Build history of the part. All positions in model axes, mm. Coordinates: 2 decimals unless noted, no trailing zeros. Loops run counter-clockwise (first coordinate to the right, second up) from the corner with the lowest first, then second, coordinate; pieces in that order, holes last. Notation, with made-up numbers: (24, -29.5) - (71, -29.5) arc R25 ccw to (71, 9.5) - close; hole circle Ø5 at (-21.75, 13). An arc over 180 degrees is marked (long way). One line per item, written item: value.
Autodesk Inventor part; units mm, degrees
ref_plane "YZ Plane" through (0, 0, 0) normal (1, 0, 0) x (0, 1, 0)
ref_plane "XZ Plane" through (0, 0, 0) normal (0, 1, 0) x (-1, 0, 0)
ref_plane "XY Plane" through (0, 0, 0) normal (0, 0, 1) x (1, 0, 0)
sketch "Sketch1" plane through (0, 0, 0) normal (1, 0, 0) x (0, 1, 0)
  line L0 (0, 0) -> (50.8, 0)
  line L1 (50.8, 0) -> (50.8, 76.2)
  line L2 (50.8, 76.2) -> (0, 76.2)
  line L3 (0, 76.2) -> (0, 0)
  dimension "d0" = 76.2
  dimension "d1" = 50.8
extrude "Extrusion1" add sketch "Sketch1" along normal blind 44.45
sketch "Sketch2" plane through (44.45, 0, 0) normal (1, 0, 0) x (0, 0, -1)
  line L0 (0, 50.8) -> (-76.2, 50.8)
  line L1 (-76.2, 50.8) -> (-76.2, 0)
  circle A0 centre (-17.272, 25.4) radius 6.35
  dimension "d4" = 12.7
  dimension "d5" = 25.4
  dimension "d6" = 58.928
extrude "Extrusion2" cut sketch "Sketch2" against normal blind 38.1
sketch "Sketch3" plane through (0, 0, 0) normal (0, 0, -1) x (-1, 0, 0)
  line L0 (0, 0) -> (0, 50.8)
  line L1 (0, 50.8) -> (-44.45, 50.8)
  line L2 (-44.45, 0) -> (-44.45, 50.8)
  line L3 (0, 0) -> (-44.45, 0)
  point P0 (-38.1, 44.45)
  point P1 (-12.7, 44.45)
  point P2 (-12.7, 6.35)
  point P3 (-38.1, 6.35)
  dimension "d9" = 6.35
  dimension "d10" = 6.35
  dimension "d11" = 6.35
  dimension "d12" = 12.7
  dimension "d13" = 12.7
  dimension "d14" = 6.35
  dimension "d15" = 6.35
  dimension "d16" = 6.35
hole "Hole1" at (38.1, 44.45, 0) at (12.7, 44.45, 0) at (12.7, 6.35, 0) at (38.1, 6.35, 0) direction (0, 0, 1) diameter 6.35 end through all
properties part number "Linear Bearing"
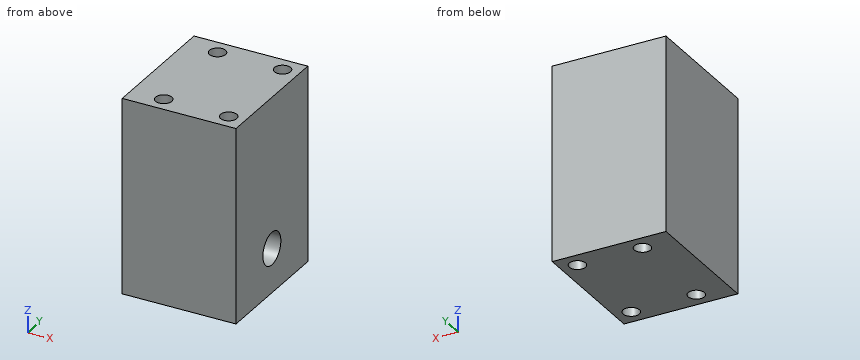
Item 1: Cut at B-B, the plane z = 47. Write the cut outline in (x, y) (3 decimals), then the cut area to 3 significant figures.
Check result:
outline: (0, 0) - (44.45, 0) - (44.45, 50.8) - (0, 50.8) - close; hole circle Ø6.35 at (12.7, 6.35); hole circle Ø6.35 at (12.7, 44.45); hole circle Ø6.35 at (38.1, 6.35); hole circle Ø6.35 at (38.1, 44.45)
area: 2,130 mm^2
Item 2: Cut at C-C, the plane y = 44.45. Write the cut outline in (x, z) (3 decimals), then the cut area to 3 significant figures.
Check result:
outline: (0, 0) - (9.525, 0) - (9.525, 76.2) - (0, 76.2) - close; (15.875, 0) - (34.925, 0) - (34.925, 76.2) - (15.875, 76.2) - close; (41.275, 0) - (44.45, 0) - (44.45, 76.2) - (41.275, 76.2) - close
area: 2,420 mm^2
Item 3: Cut at D-D, the plane x = 32. Write the cut outline in (y, z).
Check result:
outline: (0, 0) - (50.8, 0) - (50.8, 76.2) - (0, 76.2) - close; hole circle Ø12.7 at (25.4, 17.27)
Item 4: Probe probe 1 along X at (y, z) = (44.45, 27) (3 decimals); probe 2 along X at (y, z) = (47, 16); probe 3 along Y at (x, z) = (38.1, 18.5) (3 decimals). List the from-to ranges inside material, lowest first. Write a range as from..to.
Check result:
probe 1: x = 0..9.525, 15.875..34.925, 41.275..44.45
probe 2: x = 0..10.81, 14.59..36.21, 39.99..44.45
probe 3: y = 0..3.175, 9.525..19.17, 31.63..41.275, 47.625..50.8
Item 5: Cut at A-A, the plane x = 38.1. Write the cut outline in (y, z) (3 decimals).
Check result:
outline: (0, 0) - (3.175, 0) - (3.175, 76.2) - (0, 76.2) - close; (9.525, 0) - (41.275, 0) - (41.275, 76.2) - (9.525, 76.2) - close; (47.625, 0) - (50.8, 0) - (50.8, 76.2) - (47.625, 76.2) - close; hole circle Ø12.7 at (25.4, 17.272)
Item 6: Drop a flat-ended pin along its axis: P1, Ø5, axis at y = 28, z = 16, coming from the +X side. Give the stop position or say it passes through.
Check result:
P1: stops at x = 6.35
